Model file for the job. Use its own axes, mm. Face numbers are marked on the shaded views. A direction names the side the tool comes from. Coordinates: 2 decimals unless noted, no trailing zeros. Write each loop counter-clockwise with the first axis right and the second up, starting at its lowest first coordinate (ties: lowest second). Pieces come first, ordered by that corner, then holes. Notation, with made-up numbers: M -7,84.25 L 6,84.25 A25 cw 6,108.25 Z; hole C 72.25,47.5 d2. An arc over 180 degrees is marked long. Put each result on its own line as item: value. Start each with the question number.
Q1. Cut at A-A (z = 107). Write the cut outline in (x, y).
Q2. Drill centre lines: line 1 along Y through (x, z) = (545.5, 498); line 2 along Z through (x, y) = (507.5, -524). Where is each one in solid material? Low to high.
Q3. Cut at B-B (x = 83). Write the cut outline in (y, z), then the cut area to 3 significant figures.
Q4. Drop a flat-ended pin along its axis: pin 1 (10 mm diameter, centred on x = 431, z = 165, fed in from -Y). Give the stop position or say it passes through.
Q5. Cut at D-D (x = 335). Write the cut outline in (y, z), then the cut area to 3 significant figures.
Q6. Cut at C-C (z = 603). Write the cut outline in (x, y).
Q7. Which spindle directions (+Z, -Z, +X, -X, +Y, -Y) get a long thin tool onto all of the face, cutting with end or side? Do the marked faces 1 and 2. Say none if no direction does.
```python
from build123d import *

# Parameters (mm, degrees)
F0_W     = 600
F0_H     = 850
F1_DEPTH = 550
F2_SIZE2 = 80
F2_SIZE  = 25
F3_R     = 10
F4_R     = 200
F5_DEPTH = 30
F4_R_2   = 30
F6_DEPTH = 30


with BuildPart() as f1:
    # F0 (on Front) → F1 (new body)
    with BuildSketch(Plane.XZ):
        with Locations((300, 425)):
            Rectangle(F0_W, F0_H)
    extrude(amount=F1_DEPTH)

    # F2
    f2_edges = [f1.edges().sort_by_distance(p)[0] for p in [
        (300, -550, 850),
    ]]
    f2_side = f1.faces().sort_by_distance((300, -275, 850))[0]
    chamfer(f2_edges, length=F2_SIZE, length2=F2_SIZE2, reference=f2_side)

    # F3
    f3_edges = [f1.edges().sort_by_distance(p)[0] for p in [
        (0, -550, 385),
        (0, 0, 425),
        (600, -550, 385),
        (600, 0, 425),
        (0, -275, 0),
        (300, -525, 850),
        (300, -550, 770),
        (600, -262.5, 850),
        (0, -262.5, 850),
        (600, -275, 0),
        (600, -537.5, 810),
        (300, -550, 0),
        (0, -537.5, 810),
        (300, 0, 0),
        (300, 0, 850),
    ]]
    fillet(f3_edges, radius=F3_R)

    # F4 (on face) → F5 (join)
    with BuildSketch(Plane.XZ.offset(550)):
        with Locations((304.4280707836, 452.6115655899)):
            Circle(F4_R)
    extrude(amount=F5_DEPTH)

    # F4 (on face) → F6 (join)
    with BuildSketch(Plane.XZ.offset(550)):
        with Locations((532.3519706726, 724.4572639465)):
            Circle(F4_R_2)
    extrude(amount=F6_DEPTH)


solid = f1.part
```
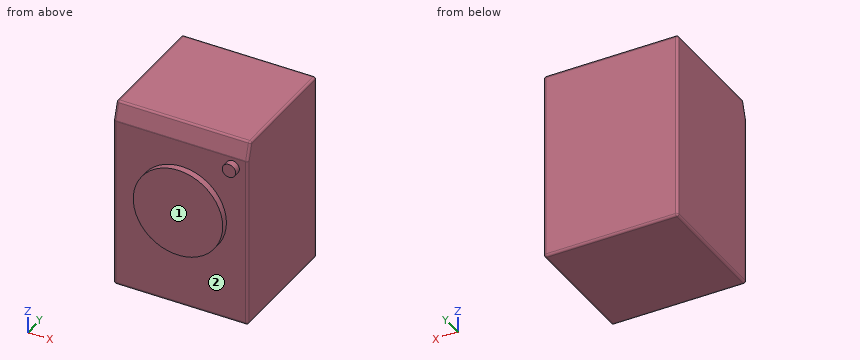
Computed values:
1. outline: M 0,-540 A10 ccw 10,-550 L 590,-550 A10 ccw 600,-540 L 600,-10 A10 ccw 590,0 L 10,0 A10 ccw 0,-10 Z
2. line 1: -550 to 0
2. line 2: 0 to 847.72
3. outline: M -550,10 A10 ccw -540,0 L -10,0 A10 ccw 0,10 L 0,840 A10 ccw -10,850 L -517.65,850 A10 ccw -527.19,842.98 L -549.54,771.46 A10 ccw -550,768.47 Z
3. area: 466,000 mm2
4. pin 1: y = -550
5. outline: M -580,254.96 L -550,254.96 L -550,10 A10 ccw -540,0 L -10,0 A10 ccw 0,10 L 0,840 A10 ccw -10,850 L -517.65,850 A10 ccw -527.19,842.98 L -549.54,771.46 A10 ccw -550,768.47 L -550,650.26 L -580,650.26 Z
5. area: 478,000 mm2
6. outline: M 0,-540 A10 ccw 10,-550 L 172.58,-550 L 172.58,-580 L 436.27,-580 L 436.27,-550 L 590,-550 A10 ccw 600,-540 L 600,-10 A10 ccw 590,0 L 10,0 A10 ccw 0,-10 Z
7. face 1: +Z, -Z, +X, -X, -Y
7. face 2: -Y
